```python
from build123d import *

# Parameters (mm, degrees)
BOSS_EXTRUDE1_DEPTH      = 32
BOSS_EXTRUDE1_DEPTH_BACK = 32
SKETCH3_R                = 20
BOSS_EXTRUDE2_DEPTH      = 8
SKETCH4_R                = 20
BOSS_EXTRUDE3_DEPTH      = 8
SKETCH5_R                = 37
BOSS_EXTRUDE4_DEPTH      = 20


with BuildPart() as part:
    # Sketch2 → Boss-Extrude1 (new body, two sides)
    with BuildSketch(Plane(origin=(0, 0, 0), x_dir=(0, 0, -1), z_dir=(1, 0, 0))) as boss_extrude1_sk:
        with BuildLine():
            Line((-11.058503278, -35.806497408), (-16.5, -41.82))
            Line((-16.5, -41.82), (-16.5, -48.82))
            Line((-16.5, -48.82), (16.5, -48.82))
            Line((16.5, -48.82), (16.5, -41.82))
            Line((16.5, -41.82), (11.058503278, -35.806497408))
            ThreePointArc((11.058503278, -35.806497408), (9.747712726, -31.031847175), (12.79921149, -27.132640587))
            ThreePointArc((12.79921149, -27.132640587), (0, 30), (-12.79921149, -27.132640587))
            ThreePointArc((-12.79921149, -27.132640587), (-9.747712726, -31.031847175), (-11.058503278, -35.806497408))
        make_face()
    extrude(amount=BOSS_EXTRUDE1_DEPTH)
    extrude(boss_extrude1_sk.sketch, amount=-BOSS_EXTRUDE1_DEPTH_BACK)

    # Sketch3 → Boss-Extrude2 (add)
    with BuildSketch(Plane(origin=(32, 0, 0), x_dir=(0, 0, -1), z_dir=(1, 0, 0))):
        Circle(SKETCH3_R)
    extrude(amount=BOSS_EXTRUDE2_DEPTH)

    # Sketch4 → Boss-Extrude3 (add)
    with BuildSketch(Plane.ZY.offset(32)):
        Circle(SKETCH4_R)
    extrude(amount=BOSS_EXTRUDE3_DEPTH)

    # Sketch5 → Boss-Extrude4 (add)
    with BuildSketch(Plane.XZ.offset(48.82)):
        Circle(SKETCH5_R)
    extrude(amount=BOSS_EXTRUDE4_DEPTH)


solid = part.part
```
Input: part model. Units: mm. Frame: model coordinates. A direction names the side the tool comes from. Give positions to 0.01 mm unless a question says otherwise; leave off trailing zeros. Order: outer loops, then holes, each group sorted by start corner. A loop starts at its lowest first (then second) coordinate and runs counter-clockwise, first axis right, second up. Notation, with made-up numbers: (25, -20.75) - (69, -20.75) arc R37 cw to (69, 17.25) - close; hole circle Ø4 at (83.25, 9). An arc over 180 degrees is marked (long way). One line per item, written item: value.
1. Cut plane C-C, the plane z = 0. Output: boundary loops of the cut face in (x, y), and give its area (3 significant figures).
Determined:
outline: (-40, -20) - (-32, -20) - (-32, -48.82) - (-37, -48.82) - (-37, -68.82) - (37, -68.82) - (37, -48.82) - (32, -48.82) - (32, -20) - (40, -20) - (40, 20) - (32, 20) - (32, 30) - (-32, 30) - (-32, 20) - (-40, 20) - close
area: 7,160 mm2
2. Cut plane D-D, the plane y = -61. Output: boundary loops of the cut face in (x, z), and give its area (3 significant figures).
Determined:
outline: circle Ø74 at (0, 0)
area: 4,300 mm2
3. Pin query (flat end, axial travel): pin 1 Ø10 at (y, z) = (-53, 1.5) entering from +X; pin 2 Ø2 at (x, z) = (-10.5, 25.5) entering from +Y; pin 3 Ø22 at (x, z) = (4.5, -16) entering from +Y; pin 4 Ø8 at (y, z) = (-38.5, -23.5) entering from +X. Return the tip coordinate at first contact, or that it passes through.
Determined:
pin 1: x = 37
pin 2: y = 17.31
pin 3: y = 29.58
pin 4: through
4. Line query: probe 1 along X at (y, z) = (-45.5, -13.5); probe 2 along Z at (x, y) = (-14.5, -44); probe 3 along Y at (x, z) = (15, 19). Output: solid intervals per line, ascending.
Determined:
probe 1: -32 to 32
probe 2: -16.5 to 16.5
probe 3: -68.82 to -48.82, -23.22 to 23.22
5. Reachability of faces 4 (the face through (-8.02, -58.68, -36.12)), 5 (the face through (-32, -18, 14)), 6 (the face through (0.45, -38.86, -13.82)), 7 (the face through (0, -45, 16.5)), 8 (the face through (32, -18, 14)) from +Z, -Z, +X, -X, +Y, -Y: full face, straight path, thin tool, end or side. Return the list, or none.
Determined:
face 4: -Y
face 5: -X
face 6: -Z, +X, -X
face 7: +Z, +X, -X
face 8: +X
6. Draft query along Y for faces 1 (the face through (0.45, 29.98, -1.13)), 2 (the face through (-1, -68.82, 1)), 3 (the face through (40, 0, 0)). Return one class per face: released by +Y, released by -Y, zero draft, split by the parting line, or undercut.
Determined:
face 1: undercut
face 2: released by -Y
face 3: zero draft
7. Cut plane B-B, the plane x = 0. Output: boundary loops of the cut face in (y, z), and give its area (3 significant figures).
Determined:
outline: (-68.82, -37) - (-48.82, -37) - (-48.82, -16.5) - (-41.82, -16.5) - (-35.81, -11.06) arc R5.51 cw to (-27.13, -12.8) arc R30 ccw (long way) to (-27.13, 12.8) arc R5.51 cw to (-35.81, 11.06) - (-41.82, 16.5) - (-48.82, 16.5) - (-48.82, 37) - (-68.82, 37) - close
area: 4,830 mm2
8. Cut plane A-A, the plane y = 0. Output: boundary loops of the cut face in (x, z), and give its area (3 significant figures).
Determined:
outline: (-40, -20) - (-32, -20) - (-32, -30) - (32, -30) - (32, -20) - (40, -20) - (40, 20) - (32, 20) - (32, 30) - (-32, 30) - (-32, 20) - (-40, 20) - close
area: 4,480 mm2
